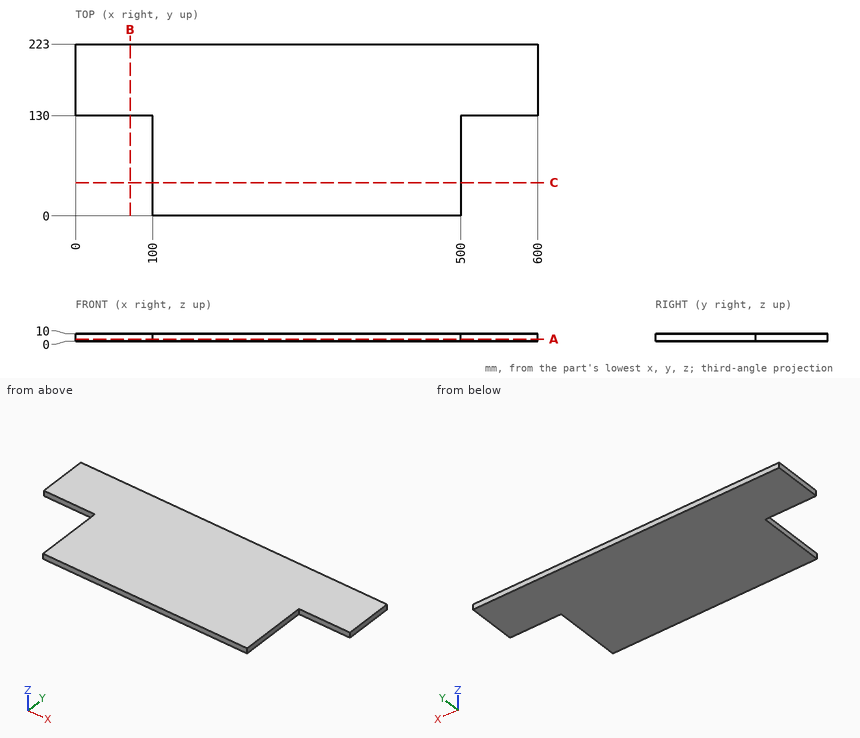
The drawing under review shows one solid part. Ordinate dimensions are in mm from its lowest x, y, z. Give positions to 0.01 mm unless a question says otherwise; leave off trailing zeros. Order: outer loops, then holes, each group sorted by start corner. A loop starts at its lowest first (then second) coordinate and runs counter-clockwise, first axis right, second up. Notation, with made-up numbers: M 43,-23 L 56,-23 A13 cw 56,-8 Z; hole C 9.25,46 d6. An arc over 180 degrees is marked long. One line per question, with ' | ' between items. Start each with the question number.
Q1. For pin 1 Ø3 at (y, z) = (85, 6.5) entering from -X; pin 2 Ø5 at (y, z) = (64.5, 3.5) entering from +X; pin 3 Ø1.5 at (x, z) = (92, 3.5) entering from -Y; pin 4 Ø1.5 at (x, y) = (466, 23.5) entering from -Z, all flat-tipped, find the tip position at first contact; note any pin that passes through.
Q2. We need section C-C (y = 43). Write out the cut boundary in (x, z), plus the area to 3 significant figures.
Q3. We need section A-A (z = 3). Write out the cut boundary in (x, y).
Q4. For L1, parallel to X at y = 9, z = 5.5; L2, parallel to Y at x = 542, z = 5.5, list the stretches that pass through material, from the lowest coordinate up. Write a range as [from, to].
Q5. We need section B-B (x = 71). Write out the cut boundary in (y, z).
Returned:
1) pin 1: x = 100 | pin 2: x = 500 | pin 3: y = 130 | pin 4: z = 0
2) outline: M 100,0 L 500,0 L 500,10 L 100,10 Z | area: 4,000 mm2
3) outline: M 0,130 L 100,130 L 100,0 L 500,0 L 500,130 L 600,130 L 600,223 L 0,223 Z
4) L1: [100, 500] | L2: [130, 223]
5) outline: M 130,0 L 223,0 L 223,10 L 130,10 Z
